```python
from build123d import *

# Parameters (mm, degrees)
BOSS_EXTRUDE1_DEPTH = 6.35
SKETCH2_R           = 14.605
CUT_EXTRUDE3_DEPTH  = 6.35
SKETCH3_R           = 8.255
CUT_EXTRUDE4_DEPTH  = 6.35
SKETCH5_R           = 1.397
CUT_EXTRUDE5_DEPTH  = 6.35


with BuildPart() as part:
    # Sketch1 → Boss-Extrude1 (new body)
    with BuildSketch(Plane.XY):
        with BuildLine():
            Line((0, 0), (38.1, 0))
            Line((38.1, 0), (38.1, -38.1))
            ThreePointArc((38.1, -38.1), (19.05, -57.15), (0, -38.1))
            Line((0, -38.1), (0, 0))
        make_face()
    extrude(amount=BOSS_EXTRUDE1_DEPTH)

    # Sketch2 → Cut-Extrude3 (cut)
    with BuildSketch(Plane.XY.offset(6.35)):
        with Locations((19.05, -38.1)):
            Circle(SKETCH2_R)
    extrude(amount=-CUT_EXTRUDE3_DEPTH, mode=Mode.SUBTRACT)

    # Sketch3 → Cut-Extrude4 (cut)
    with BuildSketch(Plane.XY.offset(6.35)):
        with Locations((19.05, -11.43)):
            Circle(SKETCH3_R)
    extrude(amount=-CUT_EXTRUDE4_DEPTH, mode=Mode.SUBTRACT)

    # Sketch5 → Cut-Extrude5 (cut)
    with BuildSketch(Plane.XY.offset(6.35)):
        with Locations((5.08, -6.35)):
            Circle(SKETCH5_R)
        with Locations((33.02, -6.35)):
            Circle(SKETCH5_R)
    extrude(amount=-CUT_EXTRUDE5_DEPTH, mode=Mode.SUBTRACT)


solid = part.part
```
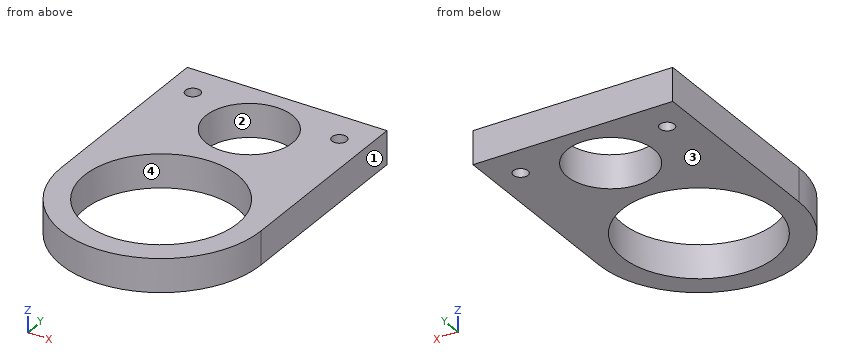
Geometry check sheet. Reference: the model listing, model coordinates, mm. Face numbers are marked on the shaded views. Give positions to 0.01 mm unless a question says otherwise; leave off trailing zeros. Order: outer loops, then holes, each group sorted by start corner. A loop starts at its lowest first (then second) coordinate and runs counter-clockwise, first axis right, second up. Notation, with made-up numbers: (20, 11.5) - (53, 11.5) arc R5 cw to (53, 16.5) - close; hole circle Ø3 at (-23.5, 24). An arc over 180 degrees is marked (long way). Write item = value, one per line. Start each with the question number.
1) Section check C-C (z = 2.25). Enter the section's corners in (x, y) (3 decimals).
2) Gauge pin test, flat ends, axial feed: pin 1 Ø4 at (x, y) = (22, -51.5) entering from +Z; pin 2 Ø1.7 at (x, y) = (33.02, -6.35) entering from -Z. Record the tip position at first contact, or that the pin passes through.
3) Section check A-A (y = -11.43). Enter the section's corners in (x, z) (3 decimals), then the cut area to 3 significant figures.
4) Section check D-D (x = 26.5). Enter the section's corners in (y, z), then the cut area to 3 significant figures.
5) Scan lines: L1, parallel to Y at x = 6, z = 1.5; L2, parallel to Y at x = 18.5, z = 5.5; L3, parallel to X at y = -19, z = 5. Record each from-to range of solid material in increasing order.
6) Section check B-B (x = 19.05). Enter the section's corners in (y, z) (3 decimals), then the cut area to 3 significant figures.
7) Draft check along X on the marked faces 1, 2, 3 and 4. Enter one of: released by +X, released by -X, zero draft, split by the parting line, or undercut.
Geometry check:
q1.outline = (0, -38.1) arc R19.05 ccw to (38.1, -38.1) - (38.1, 0) - (0, 0) - close; hole circle Ø2.794 at (5.08, -6.35); hole circle Ø29.21 at (19.05, -38.1); hole circle Ø16.51 at (19.05, -11.43); hole circle Ø2.794 at (33.02, -6.35)
q2.pin_1 = 6.35
q2.pin_2 = through
q3.outline = (0, 0) - (10.795, 0) - (10.795, 6.35) - (0, 6.35) - close; (27.305, 0) - (38.1, 0) - (38.1, 6.35) - (27.305, 6.35) - close
q3.area = 137 mm2
q4.outline = (-55.63, 0) - (-50.66, 0) - (-50.66, 6.35) - (-55.63, 6.35) - close; (-25.54, 0) - (-14.99, 0) - (-14.99, 6.35) - (-25.54, 6.35) - close; (-7.87, 0) - (0, 0) - (0, 6.35) - (-7.87, 6.35) - close
q4.area = 149 mm2
q5.L1 = -51.98 to -44.66, -31.54 to -7.4, -5.3 to 0
q5.L2 = -57.14 to -52.69, -23.51 to -19.67, -3.19 to 0
q5.L3 = 0 to 15.76, 22.34 to 38.1
q6.outline = (-57.15, 0) - (-52.705, 0) - (-52.705, 6.35) - (-57.15, 6.35) - close; (-23.495, 0) - (-19.685, 0) - (-19.685, 6.35) - (-23.495, 6.35) - close; (-3.175, 0) - (0, 0) - (0, 6.35) - (-3.175, 6.35) - close
q6.area = 72.6 mm2
q7.face_1 = released by +X
q7.face_2 = undercut
q7.face_3 = zero draft
q7.face_4 = undercut
